The listing builds one solid part. Answer for the finished solid, in the listing's coordinates (mm). Give positions to 0.01 mm unless a question says otherwise; leave off trailing zeros. Order: outer loops, then holes, each group sorted by start corner. A loop starts at its lowest first (then second) coordinate and runs counter-clockwise, first axis right, second up. Notation, with made-up numbers: (38, 82) - (77, 82) arc R26 cw to (77, 110) - close; hole circle Ø10 at (87.5, 86). An arc over 180 degrees is marked (long way). Use CSV: the item, a comma, the result in double quotes.
```python
from build123d import *

# Parameters (mm, degrees)
F0_W     = 15.875
F0_H     = 25.4
F0_W_2   = 50.8
F0_W_3   = 19.05
F1_DEPTH = 50.8


with BuildPart() as f1:
    # F0 (on Front) → F1 (new body)
    with BuildSketch(Plane.XZ):
        Polygon((336.64445, 978.200602), (336.64445, 27.277821), (349.34445, 20.754864), (349.34445, 971.677645), align=None)
        Polygon((438.24445, 926.016945), (438.24445, -24.905837), (450.94445, -31.428794), (450.94445, 919.493988), align=None)
        Polygon((539.84445, 873.833287), (539.84445, -77.089494), (552.54445, -83.612451), (552.54445, 867.31033), align=None)
        Polygon((641.44445, 821.64963), (641.44445, -129.273152), (654.14445, -135.796109), (654.14445, 815.126672), align=None)
        Polygon((743.04445, -181.456809), (755.74445, -187.979767), (755.74445, 762.943015), (743.04445, 769.465972), align=None)
        Polygon((844.64445, -233.640467), (857.34445, -240.163424), (857.34445, 710.759357), (844.64445, 717.282314), align=None)
        Polygon((946.24445, -285.824125), (958.94445, -292.347082), (958.94445, 658.5757), (946.24445, 665.098657), align=None)
        Polygon((1057.36945, -342.9), (1057.36945, -357.177219), (1057.36945, -419.1), (1076.41945, -419.1), (1076.41945, -444.5), (1057.36945, -444.5), (1057.36945, -657.225), (1108.16945, -657.225), (1108.16945, 596.208171), (1057.36945, 622.3), (1057.36945, 608.022781), align=None)
        Polygon((1057.36945, 622.3), (241.39445, 1041.4), (241.39445, 1027.122781), (336.64445, 978.200602), (349.34445, 971.677645), (438.24445, 926.016945), (450.94445, 919.493988), (539.84445, 873.833287), (552.54445, 867.31033), (641.44445, 821.64963), (654.14445, 815.126672), (743.04445, 769.465972), (755.74445, 762.943015), (844.64445, 717.282314), (857.34445, 710.759357), (946.24445, 665.098657), (958.94445, 658.5757), (1057.36945, 608.022781), align=None)
        Polygon((190.59445, 1041.4), (190.59445, 0), (241.39445, 0), (241.39445, 61.922781), (241.39445, 76.2), (241.39445, 1027.122781), (241.39445, 1041.4), align=None)
        Polygon((241.39445, 76.2), (241.39445, 61.922781), (1057.36945, -357.177219), (1057.36945, -342.9), (958.94445, -292.347082), (946.24445, -285.824125), (857.34445, -240.163424), (844.64445, -233.640467), (755.74445, -187.979767), (743.04445, -181.456809), (654.14445, -135.796109), (641.44445, -129.273152), (552.54445, -83.612451), (539.84445, -77.089494), (450.94445, -31.428794), (438.24445, -24.905837), (349.34445, 20.754864), (336.64445, 27.277821), align=None)
        Polygon((190.59445, 0), (0, 0), (0, -877.176762), (1495.213354, -877.176762), (1495.213354, -657.225), (1108.16945, -657.225), (1057.36945, -657.225), (1057.36945, -444.5), (1057.36945, -419.1), (650.96945, -419.1), (650.96945, -228.6), (650.96945, -203.2), (241.39445, -203.2), (241.39445, -25.4), (241.39445, 0), align=None)
        with Locations((658.90695, -215.9)):
            Rectangle(F0_W, F0_H)
        with Locations((266.79445, -12.7)):
            Rectangle(F0_W_2, F0_H)
        with Locations((1066.89445, -431.8)):
            Rectangle(F0_W_3, F0_H)
    extrude(amount=F1_DEPTH)


solid = f1.part
```
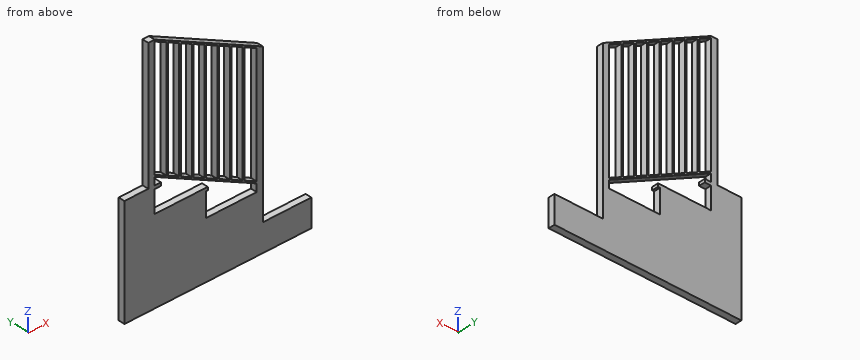
Item 1: Each of these flat-tipped pins is pushed along its axis until it touches: pin 1 (1.5 mm diameter, centred on y = -16, z = -636, fed in from +X); pin 2 (2 mm diameter, centred on x = 567.5, z = -527.5, fed in from +Y); pin 3 (15 mm diameter, centred on y = -20, z = 409, fed in from -X); pin 4 (15 mm diameter, centred on y = -37.5, z = 698, fed in from +X). Where does it stop, or does it pass through?
Taken from the geometry:
pin 1,"x = 1108.17"
pin 2,"y = 0"
pin 3,"x = 190.59"
pin 4,"x = 924.59"
Item 2: The part is cut by section A-A (x = 893). Give the vertices of the cut face in (y, z).
Taken from the geometry:
outline,"(-50.8, -877.18) - (0, -877.18) - (0, -419.1) - (-50.8, -419.1) - close; (-50.8, -272.75) - (0, -272.75) - (0, -258.48) - (-50.8, -258.48) - close; (-50.8, 692.45) - (0, 692.45) - (0, 706.72) - (-50.8, 706.72) - close"
Item 3: Find the intervals of material crossed by line 1 along Z through (x, y) = (809.5, -46.5); line 2 along Z through (x, y) = (681, -19); line 3 along X through (y, z) = (-4, 948), in increasing order.
Taken from the geometry:
line 1,"-877.18 to -419.1, -229.87 to -215.59, 735.33 to 749.61"
line 2,"-877.18 to -419.1, -163.87 to -149.59, 801.33 to 815.61"
line 3,"190.59 to 241.39, 336.64 to 349.34, 395.44 to 423.24"
Item 4: The part is cut by section D-D (z = -634). Give the vertices of the cut face in (x, y).
Taken from the geometry:
outline,"(0, -50.8) - (1108.17, -50.8) - (1108.17, 0) - (0, 0) - close"
Item 5: The part is cut by section B-B (z = 393.5). Count the separate pieces of the cut face and the enclosed holes in it, and give its area (3 significant figures).
Taken from the geometry:
separate pieces,"9"
enclosed holes,"0"
area,"9,680 mm^2"
